from build123d import *

# Parameters (mm, degrees)
SALIENTE_EXTRUIR1_DEPTH = 49
CORTAR_EXTRUIR1_DEPTH   = 70.738798384
SALIENTE_EXTRUIR3_DEPTH = 10
CROQUIS8_W              = 12
CROQUIS8_H              = 10
CORTAR_EXTRUIR2_DEPTH   = 6.5
CROQUIS9_W              = 20
CROQUIS9_H              = 12
SALIENTE_EXTRUIR4_DEPTH = 1.5


with BuildPart() as part:
    # Croquis1 → Saliente-Extruir1 (new body)
    with BuildSketch(Plane.XY):
        Polygon((-3.5, 49.5), (-3.5, 0), (0, 0), (0, 41.994225778), align=None)
    extrude(amount=SALIENTE_EXTRUIR1_DEPTH)

    # Croquis2 → Cortar-Extruir1 (cut, through all)
    with BuildSketch(Plane(origin=(0, 0, 0), x_dir=(0, 0, -1), z_dir=(1, 0, 0))):
        Polygon((-49, 0), (0, 0), (0, 28.994225778), (-14.5, 28.994225778), (-14.5, 4.5), (-34.5, 4.5), (-34.5, 28.994225778), (-49, 28.994225778), align=None)
    extrude(amount=-CORTAR_EXTRUIR1_DEPTH, mode=Mode.SUBTRACT)

    # Croquis4 → Saliente-Extruir3 (add)
    with BuildSketch(Plane.XZ.offset(-28.994225778)):
        Polygon((0, 49), (20.5, 49), (20.5, 0), (0, 0), (0, 1.5), (12.5, 1.5), (12.5, 47.5), (0, 47.5), align=None)
    extrude(amount=-SALIENTE_EXTRUIR3_DEPTH)

    # Croquis8 → Cortar-Extruir2 (cut)
    with BuildSketch(Plane(origin=(20.5, 0, 0), x_dir=(0, 0, -1), z_dir=(1, 0, 0))):
        with Locations((-24.5, 33.994225778)):
            Rectangle(CROQUIS8_W, CROQUIS8_H)
        Polygon((-48, 38.994225778), (-44.360297657, 28.994225778), (-31.590164388, 28.994225778), (-35.22986673, 38.994225778), align=None)
        Polygon((-17.409835612, 28.994225778), (-4.639702343, 28.994225778), (-1, 38.994225778), (-13.77013327, 38.994225778), align=None)
    extrude(amount=-CORTAR_EXTRUIR2_DEPTH, mode=Mode.SUBTRACT)

    # Croquis9 → Saliente-Extruir4 (add)
    with BuildSketch(Plane(origin=(0, 0, 0), x_dir=(0, 0, -1), z_dir=(1, 0, 0))):
        with Locations((-24.5, 10.5)):
            Rectangle(CROQUIS9_W, CROQUIS9_H)
    extrude(amount=SALIENTE_EXTRUIR4_DEPTH)


solid = part.part
Check sheet for the modelled part. Datum: model origin and axes. Units: mm. A direction names the side the tool comes from. Round coordinates to 2 decimals unless told otherwise and drop trailing zeros. Loops run counter-clockwise (first coordinate to the right, second up) from the corner with the lowest first, then second, coordinate; pieces in that order, holes last.
1. Scan lines: probe 1 along Z at (x, y) = (11.75, 38); probe 2 along X at (y, z) = (35, 9.5); probe 3 along X at (y, z) = (30, 18). Record each from-to range of solid material in increasing order.
2. Mould release check, pull along Z, two halves, no side actions. Record for faces 1 (the flat face through (9, 35, 0)), 2 (the flat face through (0, 32, 24)), 3 (the flat face through (20.5, 35, 17)): released by +Z, released by -Z, zero draft, split by the parting line, or undercut.
3. Sectioned sample at D-D on y = 32. Record the boundary of the cut face in (x, z).
4. Sectioned sample at A-A on z = 28. Record the boundary of the cut face in (x, y), and give its area (3 significant figures).
5. Sectioned sample at C-C on x = 9.25. Record the boundary of the cut face in (y, z).
6. Sectioned sample at B-B on x = 14.75. Record the boundary of the cut face in (y, z).
7. Set-up check for faces 4 (the flat face through (6, 34, 47.5)), 5 (the flat face through (14, 34, 25)), 6 (the flat face through (17.296, 33.924, 2.845)), 7 (the flat face through (-2, 17, 14.5)), 8 (the flat face through (17.296, 33.924, 33.385)): record each of +Z, -Z, +X, -X, +Y, -Y from which the full face is reachable in a straight line by a thin tool's end or side.
8. Gauge pin test, flat ends, axial feed: pin 1 Ø4 at (x, y) = (-1, 19) entering from -Z; pin 2 Ø3 at (y, z) = (32.5, 43.5) entering from +X; pin 3 Ø8 at (x, z) = (11, 25.5) entering from -Y; pin 4 Ø4 at (x, y) = (17.5, 25) entering from +Z. Record the tip position at first contact, or that the pin passes through.
Recorded:
1. probe 1: z = 0 to 1.5, 47.5 to 49
1. probe 2: x = -3.5 to 0, 12.5 to 14
1. probe 3: x = -3.5 to 0, 12.5 to 20.5
2. face 1: released by -Z
2. face 2: undercut
2. face 3: zero draft
3. outline: (-3.5, 0) - (20.5, 0) - (20.5, 3.55) - (14, 3.55) - (14, 16.32) - (20.5, 16.32) - (20.5, 18.5) - (14, 18.5) - (14, 30.5) - (20.5, 30.5) - (20.5, 32.68) - (14, 32.68) - (14, 45.45) - (20.5, 45.45) - (20.5, 49) - (-3.5, 49) - close; hole (0, 1.5) - (12.5, 1.5) - (12.5, 47.5) - (0, 47.5) - close
4. outline: (-3.5, 4.5) - (1.5, 4.5) - (1.5, 16.5) - (0, 16.5) - (0, 41.99) - (-3.5, 49.5) - close; (12.5, 28.99) - (14, 28.99) - (14, 38.99) - (12.5, 38.99) - close
4. area: 177 mm2
5. outline: (28.99, 0) - (38.99, 0) - (38.99, 1.5) - (28.99, 1.5) - close; (28.99, 47.5) - (38.99, 47.5) - (38.99, 49) - (28.99, 49) - close
6. outline: (28.99, 0) - (38.99, 0) - (38.99, 1) - (28.99, 4.64) - close; (28.99, 17.41) - (38.99, 13.77) - (38.99, 18.5) - (28.99, 18.5) - close; (28.99, 30.5) - (38.99, 30.5) - (38.99, 35.23) - (28.99, 31.59) - close; (28.99, 44.36) - (38.99, 48) - (38.99, 49) - (28.99, 49) - close
7. face 4: +Y, -Y
7. face 5: +X, +Y, -Y
7. face 6: +X, +Y
7. face 7: -Z, +X, -X, -Y
7. face 8: +X, -Y
8. pin 1: stops at z = 14.5
8. pin 2: stops at x = 14
8. pin 3: stops at y = 28.99
8. pin 4: passes through
